Could you check a few things on this drawing? It's one solid part, dimensions in mm from its lowest x, y, z. A direction names the side the tool comes from. Give positions to 0.01 mm unless a question says otherwise; leave off trailing zeros. Order: outer loops, then holes, each group sorted by start corner. A loop starts at its lowest first (then second) coordinate and runs counter-clockwise, first axis right, second up. Notation, with made-up numbers: M 3.5,22 L 26.5,22 A30 cw 26.5,59 Z; hole C -22.5,33 d6. An arc over 180 degrees is marked long. Use one line per item in the form item = value. Start each with the question number.
1. I want a section at C-C, the plane y = 12.75. List the corners of the cut face in (x, z) for me, and give its area (3 significant figures).
2. I want a section at B-B, the plane z = 6. List the corners of the cut face in (x, y) for me, and give its area (3 significant figures).
3. I want a section at A-A, the plane x = 8.5. List the corners of the cut face in (y, z) for me, and give its area (3 significant figures).
4. Will these pins go through, and if not, where does the flat tip stop? P1, Ø5, axis at x = 5, z = 15, coming from the +Y side; P2, Ø1.5, axis at y = 7.5, z = 17.5, coming from the -X side; P3, Ø0.9, axis at y = 8, z = 17, coming from the +X side; P4, Ø6, axis at x = 2, y = 18, coming from the -Z side.
5. I want a section at D-D, the plane z = 18.5. List the corners of the cut face in (x, y) for me, and give its area (3 significant figures).
6. For the marked faces 1, 2, 3, 4 and 5, which set-ups out of +Z, -Z, +X, -X, +Y, -Y let a thin tool reach every point of the face, with its end or its side?
7. I need wall thicknesses on L1, parallel to Y at x = 3.5, z = 9; L2, parallel to Y at x = 11.5, z = 17.75; L3, parallel to Z at x = 11.75, y = 1.5 (1 decimal). Which ranges of each line are inside material? Lowest first, please.
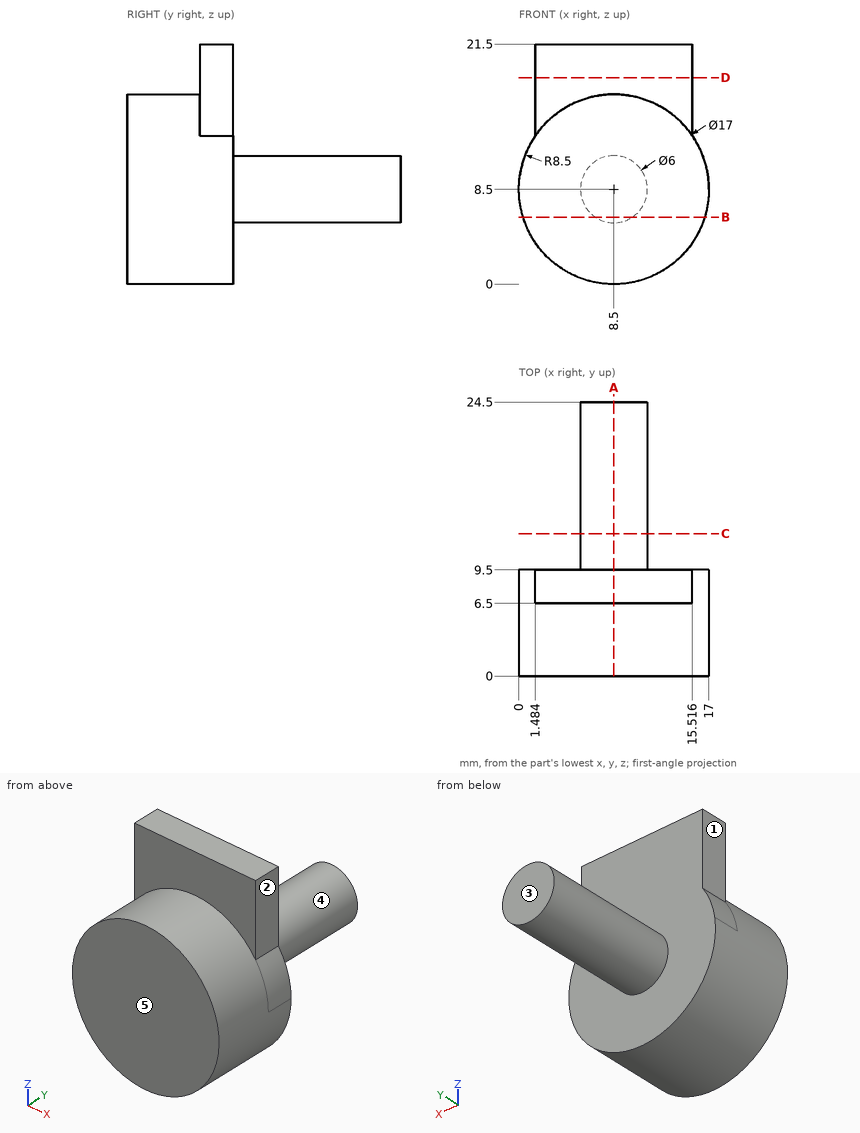
Check result:
q1.outline = C 8.5,8.5 d6
q1.area = 28.3 mm2
q2.outline = M 0.38,0 L 16.62,0 L 16.62,9.5 L 10.16,9.5 L 10.16,24.5 L 6.84,24.5 L 6.84,9.5 L 0.38,9.5 Z
q2.area = 204 mm2
q3.outline = M 0,0 L 9.5,0 L 9.5,5.5 L 24.5,5.5 L 24.5,11.5 L 9.5,11.5 L 9.5,21.5 L 6.5,21.5 L 6.5,17 L 0,17 Z
q3.area = 265 mm2
q4.P1 = 9.5
q4.P2 = 1.48
q4.P3 = 15.52
q4.P4 = through
q5.outline = M 1.48,6.5 L 15.52,6.5 L 15.52,9.5 L 1.48,9.5 Z
q5.area = 42.1 mm2
q6.face_1 = +Z, -X, +Y, -Y
q6.face_2 = +Z, +X, +Y, -Y
q6.face_3 = +Z, -Z, +X, -X, +Y
q6.face_4 = +Y
q6.face_5 = +Z, -Z, +X, -X, -Y
q7.L1 = 0 to 9.5
q7.L2 = 6.5 to 9.5
q7.L3 = 0.6 to 16.4
